For this review, use the dimensioned drawing (mm, ordinates from the lowest corner) and the shaded views. Give positions to 0.01 mm unless a question says otherwise; leave off trailing zeros. Order: outer loops, then holes, each group sorted by start corner. A loop starts at its lowest first (then second) coordinate and runs counter-clockwise, first axis right, second up.
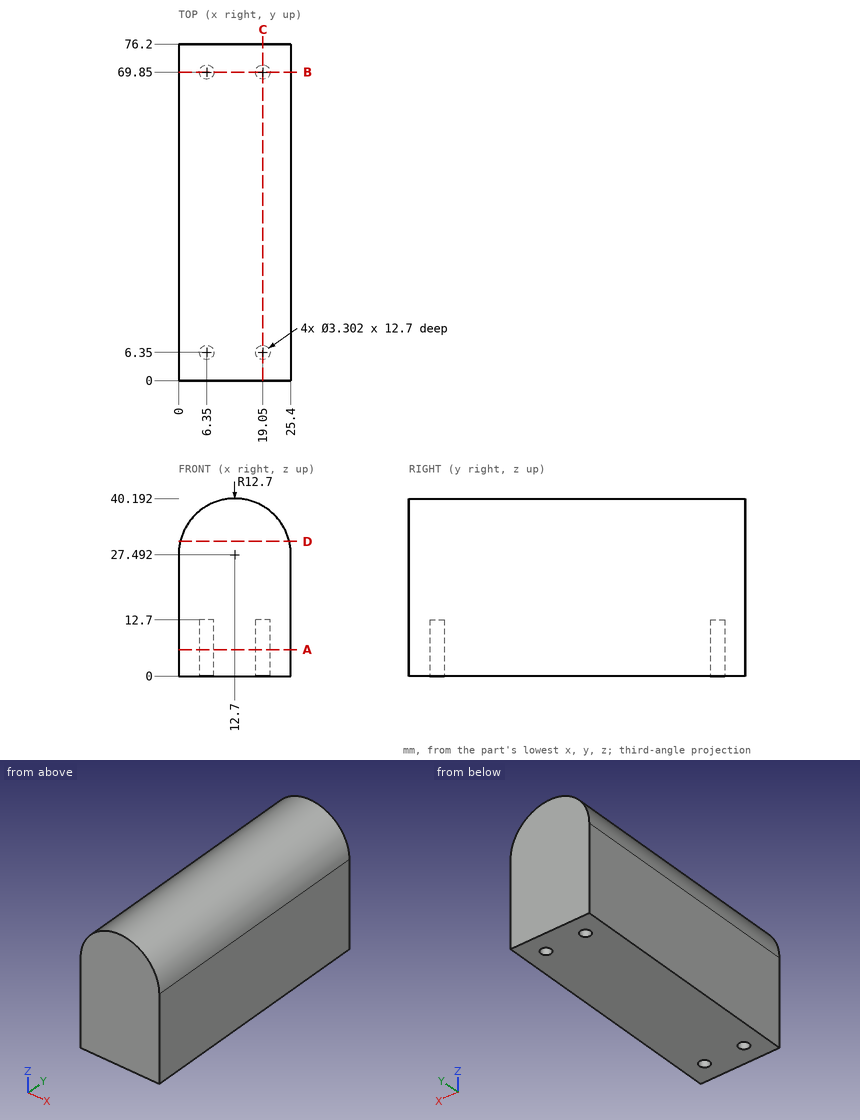
1. Take a section at C-C (x = 19.05). State the section outline as (y, z) points, then the cut area to 3 significant figures.
Recorded:
outline: (0, 0) - (4.7, 0) - (4.7, 12.7) - (8, 12.7) - (8, 0) - (68.2, 0) - (68.2, 12.7) - (71.5, 12.7) - (71.5, 0) - (76.2, 0) - (76.2, 38.49) - (0, 38.49) - close
area: 2,850 mm2
2. For pin 1 (1 mm diameter, centred on x = 19, y = 70.5, fed in from -Z); pin 2 (2 mm diameter, centred on x = 6.35, y = 6.35, fed in from +Z); pin 3 (3 mm diameter, centred on x = 21, y = 55, fed in from +Z), all flat-tipped, find the tip position at first contact; note any pin that passes through.
Recorded:
pin 1: stops at z = 12.7
pin 2: stops at z = 39.01
pin 3: stops at z = 38.22
3. Take a section at B-B (y = 69.85). State the section outline as (x, z) points, then the cut area to 3 significant figures.
Recorded:
outline: (0, 0) - (4.7, 0) - (4.7, 12.7) - (8, 12.7) - (8, 0) - (17.4, 0) - (17.4, 12.7) - (20.7, 12.7) - (20.7, 0) - (25.4, 0) - (25.4, 27.49) arc R12.7 ccw to (0, 27.49) - close
area: 868 mm2
4. Take a section at D-D (z = 30.5). State the section outline as (x, y) points, then the cut area to 3 significant figures.
Recorded:
outline: (0.36, 0) - (25.04, 0) - (25.04, 76.2) - (0.36, 76.2) - close
area: 1,880 mm2
5. For line 1 along Y through (x, z) = (19.05, 6.75); line 2 along X through (y, z) = (6, 5); line 3 along X through (y, z) = (69, 7) (1 decimal), list the stretches that pass through material, from the lowest coordinate up.
Recorded:
line 1: y = 0 to 4.7, 8 to 68.2, 71.5 to 76.2
line 2: x = 0 to 4.74, 7.96 to 17.44, 20.66 to 25.4
line 3: x = 0 to 4.9, 7.8 to 17.6, 20.5 to 25.4
6. Take a section at A-A (z = 6). State the section outline as (x, y) points.
Recorded:
outline: (0, 0) - (25.4, 0) - (25.4, 76.2) - (0, 76.2) - close; hole circle Ø3.3 at (6.35, 6.35); hole circle Ø3.3 at (6.35, 69.85); hole circle Ø3.3 at (19.05, 6.35); hole circle Ø3.3 at (19.05, 69.85)
